Can you work these out from the model? Positions are in its coordinate system, mm. Coordinates: 2 decimals unless noted, no trailing zeros. Loops run counter-clockwise (first coordinate to the right, second up) from the corner with the lowest first, then second, coordinate; pieces in that order, holes last. Notation, with made-up numbers: (-7.75, 29) - (-1.75, 29) arc R19 ccw to (-1.75, 48) - close; hole circle Ø8 at (-13.5, 20.5). An arc over 180 degrees is marked (long way). Put each result on its own line as item: value. Start each with the question number.
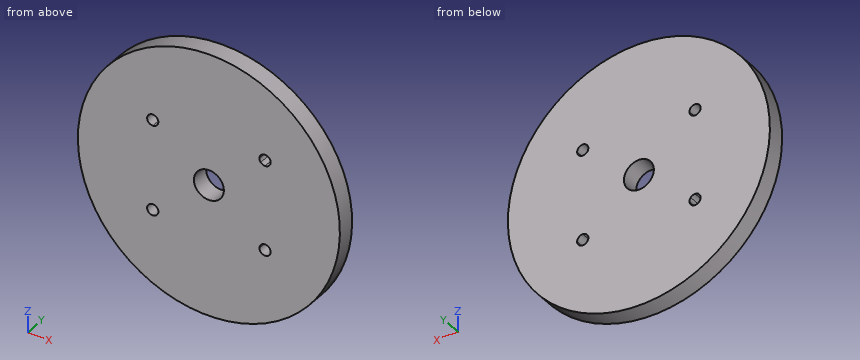
from build123d import *

# Parameters (mm, degrees)
SKETCH1_R           = 35
SKETCH1_R_2         = 4
BOSS_EXTRUDE1_DEPTH = 5
CUT_EXTRUDE1_DEPTH  = 167


with BuildPart() as part:
    # Sketch1 → Boss-Extrude1 (new body)
    with BuildSketch(Plane(origin=(0, 0, 0), x_dir=(1, 0, 0), z_dir=(0, 1, 0))):
        with Locations(Location((0, 0, 0), (0, 0, 270))):
            Circle(SKETCH1_R)
        with Locations(Location((0, 0, 0), (0, 0, 270))):
            Circle(SKETCH1_R_2, mode=Mode.SUBTRACT)
    extrude(amount=BOSS_EXTRUDE1_DEPTH)

    # Sketch2 → Cut-Extrude1 (cut)
    with BuildSketch(Plane(origin=(0, 5, 0), x_dir=(1, 0, 0), z_dir=(0, 1, 0))):
        with BuildLine():
            Line((-15, -12), (-15, -10.5))
            ThreePointArc((-15, -10.5), (-16.060660172, -13.060660172), (-13.5, -12))
            Line((-13.5, -12), (-15, -12))
        make_face()
        with BuildLine():
            ThreePointArc((-13.828696786, -11.062957429), (-14.350216904, -10.648045146), (-15, -10.5))
            Line((-15, -10.5), (-15, -12))
            Line((-15, -12), (-13.828696786, -11.062957429))
        make_face()
        with BuildLine():
            ThreePointArc((-13.5, -12), (-13.584557521, -11.503489588), (-13.828696786, -11.062957429))
            Line((-13.828696786, -11.062957429), (-15, -12))
            Line((-15, -12), (-13.5, -12))
        make_face()
        with BuildLine():
            Line((-15, 10.5), (-15, 12))
            Line((-15, 12), (-13.5, 12))
            ThreePointArc((-13.5, 12), (-16.060660172, 13.060660172), (-15, 10.5))
        make_face()
        with BuildLine():
            Line((-13.5, 12), (-15, 12))
            Line((-15, 12), (-13.828696786, 11.062957429))
            ThreePointArc((-13.828696786, 11.062957429), (-13.584557521, 11.503489588), (-13.5, 12))
        make_face()
        with BuildLine():
            Line((-13.828696786, 11.062957429), (-15, 12))
            Line((-15, 12), (-15, 10.5))
            ThreePointArc((-15, 10.5), (-14.350216904, 10.648045146), (-13.828696786, 11.062957429))
        make_face()
        with BuildLine():
            ThreePointArc((16.5, 12), (15, 13.5), (13.5, 12))
            Line((13.5, 12), (15, 12))
            Line((15, 12), (15, 10.5))
            ThreePointArc((15, 10.5), (16.060660172, 10.939339828), (16.5, 12))
        make_face()
        with BuildLine():
            Line((15, 12), (13.828696786, 11.062957429))
            ThreePointArc((13.828696786, 11.062957429), (14.350216904, 10.648045146), (15, 10.5))
            Line((15, 10.5), (15, 12))
        make_face()
        with BuildLine():
            Line((15, 12), (13.5, 12))
            ThreePointArc((13.5, 12), (13.584557521, 11.503489588), (13.828696786, 11.062957429))
            Line((13.828696786, 11.062957429), (15, 12))
        make_face()
        with BuildLine():
            Line((15, -10.5), (15, -12))
            Line((15, -12), (13.5, -12))
            ThreePointArc((13.5, -12), (15, -13.5), (16.5, -12))
            ThreePointArc((16.5, -12), (16.060660172, -10.939339828), (15, -10.5))
        make_face()
        with BuildLine():
            Line((15, -12), (13.828696786, -11.062957429))
            ThreePointArc((13.828696786, -11.062957429), (13.584557521, -11.503489588), (13.5, -12))
            Line((13.5, -12), (15, -12))
        make_face()
        with BuildLine():
            ThreePointArc((15, -10.5), (14.350216904, -10.648045146), (13.828696786, -11.062957429))
            Line((13.828696786, -11.062957429), (15, -12))
            Line((15, -12), (15, -10.5))
        make_face()
    extrude(amount=-CUT_EXTRUDE1_DEPTH, mode=Mode.SUBTRACT)


solid = part.part
Q1. Please list where these lines run through material, in increasing order: line 1 along X through (y, z) = (4.2, 0); line 2 along Z through (x, y) = (-15, 3.1); line 3 along X through (y, z) = (1.1, -12). Write a range as [from, to].
Q2. I want a section at B-B on z = 0. List the corners of the cut face in (x, y) for me.
Q3. I want a section at A-A on x = 0. List the corners of the cut face in (y, z) for me.
Q4. I want a section at C-C on y = 1. List the corners of the cut face in (x, z) for me.
Q5. Will these pins go through, and if not, where does the flat tip stop? pin 1 (1.5 mm diameter, centred on x = -11, z = -13.5, fed in from -Y); pin 2 (2 mm diameter, centred on y = 4.5, z = -7.5, fed in from +X); pin 3 (1 mm diameter, centred on y = 2.5, z = -17, fed in from -X); pin 4 (3 mm diameter, centred on x = 20, y = 3.5, fed in from -Z).
Q6. I want a section at D-D on z = 18. List the corners of the cut face in (x, y) for me, and give its area (3 significant figures).
Calculated:
1. line 1: [-35, -4], [4, 35]
1. line 2: [-31.62, -13.5], [-10.5, 10.5], [13.5, 31.62]
1. line 3: [-32.88, -16.5], [-13.5, 13.5], [16.5, 32.88]
2. outline: (-35, 0) - (-4, 0) - (-4, 5) - (-35, 5) - close; (4, 0) - (35, 0) - (35, 5) - (4, 5) - close
3. outline: (0, -35) - (5, -35) - (5, -4) - (0, -4) - close; (0, 4) - (5, 4) - (5, 35) - (0, 35) - close
4. outline: circle Ø70 at (0, 0); hole circle Ø3 at (-15, -12); hole circle Ø3 at (-15, 12); hole circle Ø8 at (0, 0); hole circle Ø3 at (15, -12); hole circle Ø3 at (15, 12)
5. pin 1: y = 0
5. pin 2: x = 34.39
5. pin 3: x = -30.87
5. pin 4: z = -29.71
6. outline: (-30.02, 0) - (30.02, 0) - (30.02, 5) - (-30.02, 5) - close
6. area: 300 mm2
